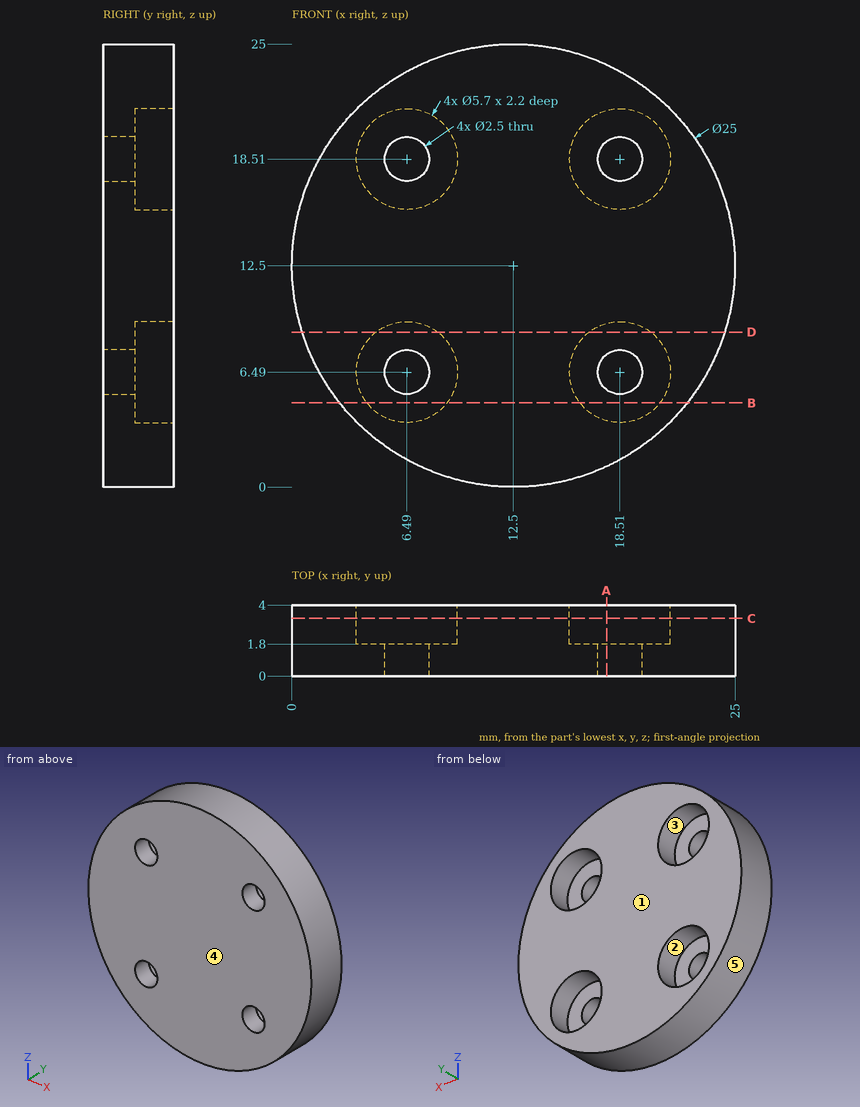
Source: three-view drawing plus pictorial views. Frame: mm from the lowest corner of the part. A direction names the side the tool comes from. Give positions to 0.01 mm unless a question says otherwise; leave off trailing zeros. Order: outer loops, then holes, each group sorted by start corner. A loop starts at its lowest first (then second) coordinate and runs counter-clockwise, first axis right, second up. Notation, with made-up numbers: M 67.5,86.5 L 117.5,86.5 A18 cw 117.5,109.5 Z; hole C -40,49 d2. An arc over 180 degrees is marked long. Return JSON: item names as keys, results as strings.
Item 1: Access query for the marked faces 1 and 2. Directions: +Z, -Z, +X, -X, +Y, -Y. A direction counts if a zero-diameter tool reaches every point of the face in a straight line with its end or side. Return the directions, or none.
Solutions:
{"face 1": "+Z, -Z, +X, -X, +Y", "face 2": "+Y"}
Item 2: Cut plane C-C (y = 3.25). Return loops of the section in (x, z), then the cut area to 3 significant figures.
Solutions:
{"outline": "C 12.5,12.5 d25; hole C 6.49,6.49 d5.7; hole C 6.49,18.51 d5.7; hole C 18.51,6.49 d5.7; hole C 18.51,18.51 d5.7", "area": "389 mm^2"}
Item 3: Ray query, probe 1 along Z at (x, y) = (6.75, 1.05); probe 2 along Z at (x, y) = (6.25, 1.6) (1 decimal); probe 3 along X at (y, z) = (1.55, 5.5) (1 decimal). Return the intervals inside material, ascending.
Solutions:
{"probe 1": "1.4 to 5.27, 7.71 to 17.29, 19.73 to 23.6", "probe 2": "1.7 to 5.3, 7.7 to 17.3, 19.7 to 23.3", "probe 3": "2.1 to 5.7, 7.3 to 17.7, 19.3 to 22.9"}
Item 4: Cut plane D-D (z = 8.75). Return loops of the section in (x, y) (1 decimal).
Solutions:
{"outline": "M 0.6,0 L 24.4,0 L 24.4,4 L 20.2,4 L 20.2,1.8 L 16.8,1.8 L 16.8,4 L 8.2,4 L 8.2,1.8 L 4.8,1.8 L 4.8,4 L 0.6,4 Z"}
Item 5: First-contact query: P1, Ø6, axis at x = 13.5, z = 11.5, coming from the -Y side; P2, Ø4.5, axis at x = 6.49, z = 6.49, coming from the +Y side. Flat tips, straight axial feed; report the tip coordinate or a pass-through.
Solutions:
{"P1": "y = 0", "P2": "y = 1.8"}
Item 6: Cut plane B-B (z = 4.75). Return loops of the section in (x, y).
Solutions:
{"outline": "M 2.69,0 L 22.31,0 L 22.31,4 L 20.77,4 L 20.77,1.8 L 16.25,1.8 L 16.25,4 L 8.75,4 L 8.75,1.8 L 4.23,1.8 L 4.23,4 L 2.69,4 Z"}
Item 7: Pull-direction query (Z, two-part tool) for the marked faces 3, 4 and 5; classes: +Z half, -Z half, draft (parallel to the pull), parting line (faces both ways), or undercut.
Solutions:
{"face 3": "undercut", "face 4": "draft", "face 5": "parting line"}
Item 8: Cut plane A-A (x = 17.75). Return loops of the section in (y, z).
Solutions:
{"outline": "M 0,1.16 L 4,1.16 L 4,3.74 L 1.8,3.74 L 1.8,5.5 L 0,5.5 Z; M 0,7.48 L 1.8,7.48 L 1.8,9.24 L 4,9.24 L 4,15.76 L 1.8,15.76 L 1.8,17.52 L 0,17.52 Z; M 0,19.5 L 1.8,19.5 L 1.8,21.26 L 4,21.26 L 4,23.84 L 0,23.84 Z"}
